Source: CAD feature listing. Evaluate the final solid. Frame: model axes, mm. Face numbers are marked on the shaded views. A direction names the side the tool comes from. Give positions to 0.01 mm unless a question says otherwise; leave off trailing zeros. Order: outer loops, then holes, each group sorted by start corner. A loop starts at its lowest first (then second) coordinate and runs counter-clockwise, first axis right, second up. Notation, with made-up numbers: M -11,22 L 26,22 A15 ccw 26,41 Z; hole C 81.25,42 d4. An arc over 180 degrees is marked long. Use CSV: the item, a comma, the result in double quotes. Start each with the question number.
Item 1: Ray query, probe 1 along Y at (x, z) = (0, 18); probe 2 along X at (y, z) = (-45, 34.25); probe 3 along Y at (x, z) = (0, 34). Return the intervals inside material, ascending. Write a range as from..to.
Item 2: First-contact query: pin 1 (1.5 mm diameter, centred on x = -21.5, z = 33, fed in from +Y); pin 2 (4 mm diameter, centred on x = 13.5, z = 37, fed in from +Y); pin 3 (18 mm diameter, centred on x = 5, y = -4, fed in from +Z). Flat tips, straight axial feed; report the tip coordinate or a pass-through.
Item 3: Section query B-B on y = -55.5. Return loops of the section in (x, z).
Item 4: Section query C-C on z = 20. Return loops of the section in (x, y), and give its area (3 significant figures).
Item 5: Section query D-D on x = -11.5. Return loops of the section in (y, z).
Item 6: Section query A-A on x = 0. Return loops of the section in (y, z), and give its area (3 significant figures).
Item 7: Access query for the marked faces 1 and 2. Directions: +Z, -Z, +X, -X, +Y, -Y. A direction counts if a zero-diameter tool reaches every point of the face in a straight line with its end or side. Return the directions, or none.
from build123d import *

# Parameters (mm, degrees)
F0_R     = 15
F1_DEPTH = 25
F2_R     = 15
F3_DEPTH = 50


with BuildPart() as f1:
    # F0 (on Top) → F1 (new body)
    with BuildSketch(Plane.XY):
        with BuildLine():
            Line((30, -45), (30, 45))
            Line((30, 45), (-30, 45))
            Line((-30, 45), (-30, -45))
            ThreePointArc((-30, -45), (0, -15), (30, -45))
        make_face()
        with BuildLine():
            ThreePointArc((-30, -45), (0, -75), (30, -45))
            ThreePointArc((30, -45), (0, -15), (-30, -45))
        make_face()
        with Locations((0, -45)):
            Circle(F0_R, mode=Mode.SUBTRACT)
    extrude(amount=F1_DEPTH)

    # F2 (on face) → F3 (join)
    with BuildSketch(Plane(origin=(0, 0, 0), x_dir=(1, 0, 0), z_dir=(0, 0, -1))):
        with BuildLine():
            ThreePointArc((30, 45), (0, 75), (-30, 45))
            ThreePointArc((-30, 45), (0, 15), (30, 45))
        make_face()
        with Locations((0, 45)):
            Circle(F2_R, mode=Mode.SUBTRACT)
    extrude(amount=-F3_DEPTH)


solid = f1.part
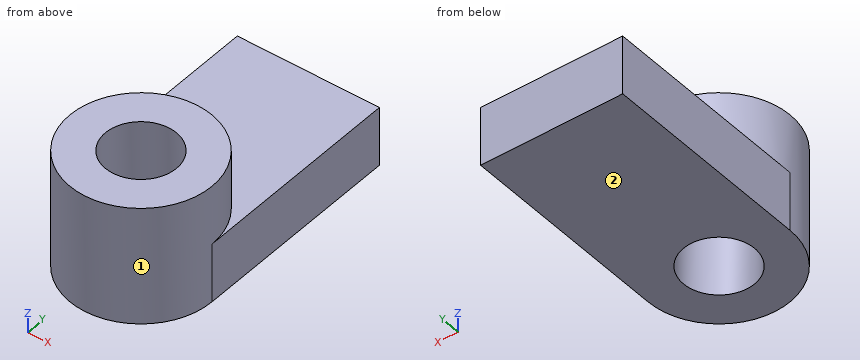
Verdict:
1,probe 1,"-75..-60, -30..45"
1,probe 2,"-30..-15, 15..30"
1,probe 3,"-75..-60, -30..-15"
2,pin 1,"y = -23.33"
2,pin 2,"y = -17.29"
2,pin 3,"z = 25"
3,outline,"M -28.1,0 L -10.71,0 L -10.71,50 L -28.1,50 Z; M 10.71,0 L 28.1,0 L 28.1,50 L 10.71,50 Z"
4,outline,"M -30,-45 A30 ccw 30,-45 L 30,45 L -30,45 Z; hole C 0,-45 d30"
4,area,"6,110 mm2"
5,outline,"M -72.71,0 L -54.63,0 L -54.63,50 L -72.71,50 Z; M -35.37,0 L 45,0 L 45,25 L -17.29,25 L -17.29,50 L -35.37,50 Z"
6,outline,"M -75,0 L -60,0 L -60,50 L -75,50 Z; M -30,0 L 45,0 L 45,25 L -15,25 L -15,50 L -30,50 Z"
6,area,"3,000 mm2"
7,face 1,"+Z"
7,face 2,"-Z, +X, -X, +Y, -Y"
